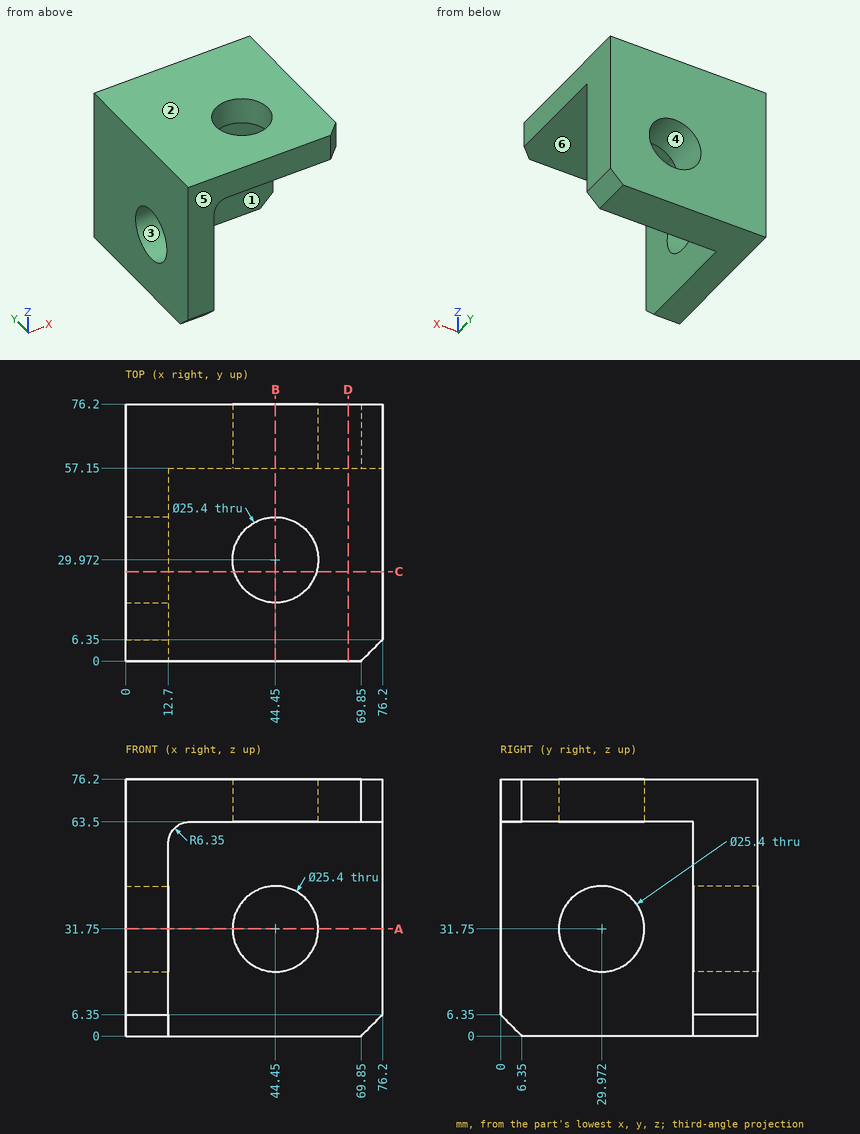
Geometry: see drawing. Coordinates: mm, zero at the bounding-box minimum. A direction names the side the tool comes from. Round coordinates to 2 decimals unless told otherwise and drop trailing zeros. Loops run counter-clockwise (first coordinate to the right, second up) from the corner with the lowest first, then second, coordinate; pieces in that order, holes last. Notation, with made-up numbers: (-6, -18.75) - (4, -18.75) arc R14 ccw to (4, -2.75) - close; hole circle Ø11 at (10.25, -24). An arc over 180 degrees is marked (long way). Use CSV: the item, a comma, the result in double quotes.
Q1. Section query B-B, the plane x = 44.45. Output: boundary loops of the cut face in (y, z).
Reported:
outline,"(0, 63.5) - (17.27, 63.5) - (17.27, 76.2) - (0, 76.2) - close; (42.67, 63.5) - (57.15, 63.5) - (57.15, 44.45) - (76.2, 44.45) - (76.2, 76.2) - (42.67, 76.2) - close; (57.15, 0) - (76.2, 0) - (76.2, 19.05) - (57.15, 19.05) - close"
Q2. Mould query, pull axis Z, two halves, no side actions, for the marked faces 3, 4, 5 and 6. Classes: pulls with the +Z half, pulls with the -Z half, needs draft (parallel to the pull), parting line crosses it, or undercut.
Reported:
face 3,"undercut"
face 4,"undercut"
face 5,"needs draft"
face 6,"pulls with the -Z half"
Q3. Pin query (flat end, axial travel): pin 1 Ø5 at (y, z) = (37.5, 41.5) entering from +X; pin 2 Ø19 at (x, z) = (42.5, 36) entering from -Y; pin 3 Ø3 at (y, z) = (52, 59) entering from -X; pin 4 Ø23 at (x, z) = (44.45, 31.75) entering from -Y. Return the tip coordinate at first contact, or that it passes through.
Reported:
pin 1,"x = 12.7"
pin 2,"y = 57.15"
pin 3,"x = 0"
pin 4,"through"
Q4. Section query A-A, the plane z = 31.75. Output: boundary loops of the cut face in (x, y), then the cut area to 3 significant figures.
Reported:
outline,"(0, 0) - (12.7, 0) - (12.7, 17.27) - (0, 17.27) - close; (0, 42.67) - (12.7, 42.67) - (12.7, 57.15) - (31.75, 57.15) - (31.75, 76.2) - (0, 76.2) - close; (57.15, 57.15) - (76.2, 57.15) - (76.2, 76.2) - (57.15, 76.2) - close"
area,"1,370 mm^2"
Q5. Ray query, line 1 along Y through (x, z) = (2, 31); line 2 along Z through (x, y) = (44.45, 66.25); line 3 along Y through (x, z) = (44, 73). Return the intervals inside material, ascending.
Reported:
line 1,"0 to 17.29, 42.65 to 76.2"
line 2,"0 to 19.05, 44.45 to 76.2"
line 3,"0 to 17.28, 42.66 to 76.2"
Q6. Section query C-C, the plane y = 26.5. Output: boundary loops of the cut face in (x, z).
Reported:
outline,"(0, 0) - (12.7, 0) - (12.7, 19.53) - (0, 19.53) - close; (0, 43.97) - (12.7, 43.97) - (12.7, 57.15) arc R6.35 cw to (19.05, 63.5) - (32.23, 63.5) - (32.23, 76.2) - (0, 76.2) - close; (56.67, 63.5) - (76.2, 63.5) - (76.2, 76.2) - (56.67, 76.2) - close"
Q7. Reachability of the marked faces 1 and 2 from +Z, -Z, +X, -X, +Y, -Y: full face, straight path, thin tool, end or side. Return the list, or none.
Reported:
face 1,"-Z, +X, -Y"
face 2,"+Z, +X, -X, +Y, -Y"
Q8. Section query D-D, the plane x = 66. Output: boundary loops of the cut face in (y, z).
Reported:
outline,"(0, 63.5) - (57.15, 63.5) - (57.15, 0) - (76.2, 0) - (76.2, 76.2) - (0, 76.2) - close"
